Input: part model. Units: mm. Frame: model coordinates. A direction names the side the tool comes from. Coordinates: 2 decimals unless noted, no trailing zeros. Order: outer loops, then holes, each group sorted by start corner. A loop starts at its lowest first (then second) coordinate and runs counter-clockwise, first axis right, second up. Notation, with made-up numbers: M 21.25,65 L 58.25,65 A13 ccw 58.25,89 Z; hole C 29,52 d9. An arc over 180 degrees is marked long. Answer in a Markdown table with one row per item.
from build123d import *

# Parameters (mm, degrees)
SKETCH1_R           = 9.525
BOSS_EXTRUDE1_DEPTH = 25.4
SKETCH4_R           = 9.525
SKETCH4_R_2         = 6.35
CUT_EXTRUDE1_DEPTH  = 12.7


with BuildPart() as part:
    # Sketch1 → Boss-Extrude1 (new body)
    with BuildSketch(Plane.XY):
        Circle(SKETCH1_R)
    extrude(amount=BOSS_EXTRUDE1_DEPTH)

    # Cut-Loft1: read off the stored shape, not the designer's step
    # Cut-Loft1: loft between two sections, ruled curve by curve
    cut_loft1_from = [
        Edge.make_bspline([(4.189007655, 2.396349487, 25.4), (8.981706629, -5.981665824, 25.4), (0.603691318, -10.774364798, 25.4), (-4.189007655, -2.396349487, 25.4), (-8.981706629, 5.981665824, 25.4), (-0.603691318, 10.774364798, 25.4), (4.189007655, 2.396349487, 25.4)], [0, 0, 0, 0, 0.5, 0.5, 0.5, 1, 1, 1, 1], 3, [1, 0.333333333, 0.333333333, 1, 0.333333333, 0.333333333, 1]),
    ]
    cut_loft1_to = [
        Edge.make_bspline([(2.245993729, 0.791115497, 0), (3.828224724, -3.700871962, 0), (-0.663762735, -5.283102956, 0), (-2.245993729, -0.791115497, 0), (-3.828224724, 3.700871962, 0), (0.663762735, 5.283102956, 0), (2.245993729, 0.791115497, 0)], [0, 0, 0, 0, 0.5, 0.5, 0.5, 1, 1, 1, 1], 3, [1, 0.333333333, 0.333333333, 1, 0.333333333, 0.333333333, 1]),
    ]
    cut_loft1 = Solid(Shell([*[Face.make_surface_from_curves(cut_loft1_from[k], cut_loft1_to[k]) for k in range(1)], Face(Wire(cut_loft1_from)), Face(Wire(cut_loft1_to))]))
    add(cut_loft1, mode=Mode.SUBTRACT)

    # Sketch4 → Cut-Extrude1 (cut)
    with BuildSketch(Plane(origin=(0, 0, 0), x_dir=(-1, 0, 0), z_dir=(0, 0, -1))):
        Circle(SKETCH4_R)
        Circle(SKETCH4_R_2, mode=Mode.SUBTRACT)
    extrude(amount=-CUT_EXTRUDE1_DEPTH, mode=Mode.SUBTRACT)


solid = part.part
1) Reachability of faces 1 (the face through (1.38, -6.2, 6.26)), 2 (the face through (-2, -5, 25.4)) from +Z, -Z, +X, -X, +Y, -Y: full face, straight path, thin tool, end or side. Return the list, or none.
Resolved:
| item | result |
|---|---|
| face 1 | -Z |
| face 2 | +Z, +X, -X, +Y, -Y |
2) Material intervals for probe 1 along Z at (x, y) = (-2.25, -8); probe 2 along Y at (x, z) = (0.5, 8); probe 3 along Y at (x, z) = (-0.5, 22.5), sorted ascending.
Resolved:
| item | result |
|---|---|
| probe 1 | z = 12.7 to 25.4 |
| probe 2 | y = -6.33 to -3.1, 3.1 to 6.33 |
| probe 3 | y = -9.51 to -4.52, 4.52 to 9.51 |
3) Cut plane A-A, the plane x = 5.25. Output: boundary loops of the cut face in (y, z), and give its area (3 significant figures).
Resolved:
| item | result |
|---|---|
| outline | M -7.95,12.7 L -3.57,12.7 L -3.57,0 L 3.57,0 L 3.57,12.7 L 7.95,12.7 L 7.95,25.4 L -7.95,25.4 Z |
| area | 293 mm2 |
4) Contact query for flat-ended pins moving along their axis: pin 1 (5 mm diameter, centred on y = -4, z = 6.5, fed in from +X); pin 2 (4 mm diameter, centred on x = -3, z = 7.5, fed in from -Y); pin 3 (3 mm diameter, centred on x = -3, z = 22, fed in from +Y). Output: stop coordinate, or through.
Resolved:
| item | result |
|---|---|
| pin 1 | stops at x = 6.17 |
| pin 2 | stops at y = -6.27 |
| pin 3 | stops at y = 9.41 |
5) Cut plane C-C, the plane y = -6.75. Output: boundary loops of the cut face in (x, z).
Resolved:
| item | result |
|---|---|
| outline | M -6.72,12.7 L 6.72,12.7 L 6.72,25.4 L -6.72,25.4 Z |
6) Cut plane B-B, the plane x = -5.5. Output: boundary loops of the cut face in (y, z).
Resolved:
| item | result |
|---|---|
| outline | M -7.78,12.7 L -3.17,12.7 L -3.17,0 L 3.17,0 L 3.17,12.7 L 7.78,12.7 L 7.78,25.4 L -7.78,25.4 Z |
